Source: CAD feature listing. Evaluate the final solid. Frame: model axes, mm. A direction names the side the tool comes from. Round coordinates to 2 decimals unless told otherwise and drop trailing zeros. Order: outer loops, then holes, each group sorted by start corner. A loop starts at its lowest first (then second) coordinate and runs counter-clockwise, first axis right, second up. Notation, with made-up numbers: M -28,35 L -8,35 A25 cw -8,49 Z; hole C 72.5,36 d11. An arc over 180 degrees is marked long. Answer in a Markdown table with one row per item. Add a question column.
```python
from build123d import *

# Parameters (mm, degrees)
F0_W          = 50.8
F0_H          = 50.8
F1_DEPTH      = 3.175
F2_W          = 50.8
F2_H          = 3.175
F3_DEPTH      = 12.7
F3_DEPTH_BACK = 76.2
F4_W          = 3.175
F4_H          = 101.6
F5_DEPTH      = 12.7
F5_DEPTH_BACK = 76.2
F7_W          = 47.625
F7_H          = 12.7
F8_DEPTH      = 25.4
F9_W          = 47.625
F9_H          = 12.7
F10_DEPTH     = 25.4
F12_DEPTH     = 25.4
F14_DEPTH     = 25.4
F16_DEPTH     = 53.976
F18_DEPTH     = 76.2
F19_R         = 3.175
F20_DEPTH     = 25.4
F21_R         = 3.175
F22_DEPTH     = 25.4
F23_R         = 3.175
F24_DEPTH     = 25.4
F26_DEPTH     = 76.201
F27_DEPTH     = 3.175
F29_DEPTH     = 76.2
F31_DEPTH     = 76.201
F32_W         = 3.175
F32_H         = 76.2
F33_DEPTH     = 12.7
F35_DEPTH     = 25.4


with BuildPart() as f1:
    # F0 (on Top) → F1 (new body)
    with BuildSketch(Plane.XY):
        with Locations((25.4, 25.4)):
            Rectangle(F0_W, F0_H)
    extrude(amount=F1_DEPTH)

    # F2 (on face) → F3 (join, two sides)
    with BuildSketch(Plane.XY.offset(3.175)) as f3_sk:
        with Locations((-25.4, 1.5875)):
            Rectangle(F2_W, F2_H)
        with Locations((25.4, 1.5875)):
            Rectangle(F2_W, F2_H)
    extrude(amount=F3_DEPTH)
    extrude(f3_sk.sketch, amount=-F3_DEPTH_BACK)

    # F4 (on face) → F5 (join, two sides)
    with BuildSketch(Plane.XY.offset(3.175)) as f5_sk:
        with Locations((1.5875, 0)):
            Rectangle(F4_W, F4_H)
    extrude(amount=F5_DEPTH)
    extrude(f5_sk.sketch, amount=-F5_DEPTH_BACK)

    # F7 (on face) → F8 (cut)
    with BuildSketch(Plane.YZ.offset(3.175)):
        with Locations((26.9875, 9.525)):
            Rectangle(F7_W, F7_H)
    extrude(amount=-F8_DEPTH, mode=Mode.SUBTRACT)

    # F9 (on face) → F10 (cut)
    with BuildSketch(Plane(origin=(0, 3.175, 0), x_dir=(-1, 0, 0), z_dir=(0, 1, 0))):
        with Locations((-26.9875, 9.525)):
            Rectangle(F9_W, F9_H)
    extrude(amount=-F10_DEPTH, mode=Mode.SUBTRACT)

    # F11 (on face) → F12 (cut)
    with BuildSketch(Plane.XZ):
        Polygon((50.8, -6.35), (41.275, -73.025), (50.8, -73.025), align=None)
    extrude(amount=-F12_DEPTH, mode=Mode.SUBTRACT)

    # F13 (on face) → F14 (cut)
    with BuildSketch(Plane(origin=(0, 0, 0), x_dir=(0, -1, 0), z_dir=(-1, 0, 0))):
        Polygon((-15.875, -73.025), (-50.8, -6.35), (-50.8, -73.025), align=None)
    extrude(amount=-F14_DEPTH, mode=Mode.SUBTRACT)

    # F15 (on face) → F16 (cut, through all)
    with BuildSketch(Plane(origin=(0, 3.175, 0), x_dir=(-1, 0, 0), z_dir=(0, 1, 0))):
        Polygon((50.8, 15.875), (-3.175, 15.875), (-3.175, 3.175), (0, 3.175), (50.8, 3.175), align=None)
    extrude(amount=-F16_DEPTH, mode=Mode.SUBTRACT)

    # F17 (on face) → F18 (join, through all)
    with BuildSketch(Plane.XY.offset(3.175)):
        Polygon((9.525, 0), (3.175, 0), (3.175, -6.35), align=None)
        Polygon((-6.35, 3.175), (0, 3.175), (0, 9.525), align=None)
    extrude(amount=-F18_DEPTH)

    # F19 (on face) → F20 (cut)
    with BuildSketch(Plane(origin=(0, 3.175, 0), x_dir=(-1, 0, 0), z_dir=(0, 1, 0))):
        with Locations((-26.9875, -12.7)):
            Circle(F19_R)
    extrude(amount=-F20_DEPTH, mode=Mode.SUBTRACT)

    # F21 (on face) → F22 (cut)
    with BuildSketch(Plane.YZ.offset(3.175)):
        with Locations((26.9875, -12.7)):
            Circle(F21_R)
    extrude(amount=-F22_DEPTH, mode=Mode.SUBTRACT)

    # F23 (on face) → F24 (cut)
    with BuildSketch(Plane(origin=(0, 0, 0), x_dir=(1, 0, 0), z_dir=(0, 0, -1))):
        with Locations((26.9875, -26.9875)):
            Circle(F23_R)
    extrude(amount=-F24_DEPTH, mode=Mode.SUBTRACT)

    # F25 (on face) → F26 (cut, through all)
    with BuildSketch(Plane.XY.offset(3.175)):
        Polygon((41.275, 0), (50.8, 0), (50.8, 50.8), (41.275, 50.8), (0, 50.8), (0, 41.275), (41.275, 41.275), align=None)
    extrude(amount=-F26_DEPTH, mode=Mode.SUBTRACT)

    # F27 (add): a face of the model
    f27_faces = [f1.faces().sort_by_distance(p)[0] for p in [
        (-25.4, 0, -34.925),
    ]]
    extrude(f27_faces, amount=F27_DEPTH)

    # F28 (on face) → F29 (join, through all)
    with BuildSketch(Plane.XY.offset(3.175)):
        Polygon((28.575, 0), (22.225, 0), (19.05, 0), (19.05, -50.8), (22.225, -50.8), (22.225, -6.35), align=None)
    extrude(amount=-F29_DEPTH)

    # F30 (on face) → F31 (cut, through all)
    with BuildSketch(Plane.XY.offset(3.175)):
        Polygon((0, -50.8), (3.175, -50.8), (3.175, -6.35), (6.35, -3.175), (0, -3.175), align=None)
    extrude(amount=-F31_DEPTH, mode=Mode.SUBTRACT)

    # F32 (on face) → F33 (join, through all)
    with BuildSketch(Plane(origin=(19.05, 0, 0), x_dir=(0, -1, 0), z_dir=(-1, 0, 0))):
        with Locations((1.5875, -34.925)):
            Rectangle(F32_W, F32_H)
    extrude(amount=F33_DEPTH)

    # F34 (on face) → F35 (join)
    with BuildSketch(Plane(origin=(0, 0, -73.025), x_dir=(1, 0, 0), z_dir=(0, 0, -1))):
        Polygon((19.05, 3.175), (6.35, 3.175), (-50.8, 3.175), (-50.8, -3.175), (-6.35, -3.175), (0, -9.525), (0, -15.875), (3.175, -15.875), (3.175, -3.175), (41.275, -3.175), (41.275, 0), (28.575, 0), (22.225, 6.35), (22.225, 50.8), (19.05, 50.8), align=None)
    extrude(amount=F35_DEPTH)


solid = f1.part
```
(1) Cut plane B-B (z = -53). Return loops of the section in (x, y) (3 decimals).
(2) Cut plane C-C (y = -10.5). Return loops of the section in (x, z) (3 decimals).
(3) Draft query along X for faces 1 (the face through (22, 22, 0)), 2 (the face through (24.47, 28.92, 1.57)), 3 (the face through (19.05, -27, -47)). Return one class per face: +X half, -X half, draft (parallel to the pull), parting line (faces both ways), or undercut.
(4) Line query: line 1 (X direction, y = 27.5, z = -18) (3 decimals); line 2 (Y direction, x = -23.5, z = -57.5) (3 decimals); line 3 (X direction, y = -7.5, z = -36) (3 decimals). Output: solid intervals per line, ascending. Write a range as from..to.
(5) Cut plane D-D (x = -9). Return loops of the section in (y, z) (3 decimals).
(6) Access query for faces 4 (the face through (-15, -3.175, -47)), 5 (the face through (0, 22, -36)), 6 (the face through (29.51, 1.61, -14.63)). Directions: +Z, -Z, +X, -X, +Y, -Y. A direction counts if a zero-diameter tool reaches every point of the face in a straight line with its end or side. Return the directions, or none.
(7) Pin query (flat end, axial travel): pin 1 (8.5 mm diameter, centred on y = 26.99, z = -12.7, fed in from +X) (3 decimals); pin 2 (7.5 mm diameter, centred on x = 26.99, y = 26.99, fed in from -Z); pin 3 (1 mm diameter, centred on x = 1.5, z = -89.5, fed in from +Y) (3 decimals); pin 4 (11.5 mm diameter, centred on y = 28, z = -69, fed in from +X). Return the tip coordinate at first contact, or that it passes through.
(8) Cut plane A-A (z = -12.7). Count the separate pieces of the cut face and the enclosed holes in it, and give its area (3 significant figures).
Answer list:
| question | item | result |
|---|---|---|
| 1 | outline | M -50.8,-3.175 L 19.05,-3.175 L 19.05,-50.8 L 22.225,-50.8 L 22.225,-6.35 L 28.575,0 L 41.275,0 L 41.275,3.175 L 3.175,3.175 L 3.175,26.364 L 0,26.364 L 0,9.525 L -6.35,3.175 L -50.8,3.175 Z |
| 2 | outline | M 19.05,-98.425 L 22.225,-98.425 L 22.225,3.175 L 19.05,3.175 Z |
| 3 | face 1 | draft |
| 3 | face 2 | undercut |
| 3 | face 3 | -X half |
| 4 | line 1 | 0..3.175 |
| 4 | line 2 | -3.175..3.175 |
| 4 | line 3 | 19.05..22.225 |
| 5 | outline | M -3.175,-98.425 L 3.175,-98.425 L 3.175,3.175 L -3.175,3.175 Z |
| 6 | face 4 | +Z, -Z, -X, -Y |
| 6 | face 5 | +Z, -Z, -X, +Y |
| 6 | face 6 | +Y |
| 7 | pin 1 | x = 3.175 |
| 7 | pin 2 | z = 0 |
| 7 | pin 3 | y = 15.875 |
| 7 | pin 4 | through |
| 8 | separate pieces | 3 |
| 8 | enclosed holes | 0 |
| 8 | area | 796 mm² |
